```python
from build123d import *

# Parameters (mm, degrees)
BOSS_EXTRUDE1_DEPTH            = 1.6
F_2_2_2_2_DIAMETER_HOLE1_D     = 2.2
F_2_2_2_2_DIAMETER_HOLE1_DEPTH = 5
SKETCH9_R                      = 10
CUT_EXTRUDE4_DEPTH             = 2.6
SKETCH15_W                     = 83
SKETCH15_H                     = 2.5
CUT_EXTRUDE8_DEPTH             = 2.6
SKETCH37_W                     = 83
SKETCH37_H                     = 1.6
EXTRUDE1_DEPTH                 = 1.6
SKETCH38_W                     = 83
SKETCH38_H                     = 1.6
EXTRUDE2_DEPTH                 = 1.6
F_2_2_2_2_DIAMETER_HOLE4_D     = 2.2
F_2_2_2_2_DIAMETER_HOLE4_DEPTH = 1.6
SKETCH49_W                     = 0.2
SKETCH49_H                     = 100.7
EXTRUDE5_DEPTH                 = 2.6
SKETCH51_W                     = 10
SKETCH51_H                     = 10
CUT_EXTRUDE9_DEPTH             = 10
SKETCH52_W                     = 19
SKETCH52_H                     = 6.1
CUT_EXTRUDE10_DEPTH            = 2.6
SKETCH_2_R                     = 1.6
CUT_EXTRUDE_2_DEPTH            = 10
SKETCH_8_R                     = 0.3
CUT_EXTRUDE_3_DEPTH            = 10
SKETCH_9_R                     = 1.1
CUT_EXTRUDE_4_DEPTH            = 10
SKETCH_10_R                    = 2
CUT_EXTRUDE_5_DEPTH            = 0.01
SKETCH_11_R                    = 1.1
CUT_EXTRUDE_6_DEPTH            = 10


with BuildPart() as part:
    # Sketch1 → Boss-Extrude1 (new body)
    with BuildSketch(Plane(origin=(0, 0, 0), x_dir=(1, 0, 0), z_dir=(0, 1, 0))):
        Polygon((65.24, 0.272495156), (65.24, -46.437452638), (65.24, -63.637452638), (65.24, -70.137452638), (-17.76, -70.137452638), (-17.76, -63.637452638), (-17.76, -48.637452638), (-17.76, -45.78978272), (-17.76, 4.362547362), (-17.76, 21.562547362), (-17.76, 29.862547362), (65.24, 29.862547362), (65.24, 21.562547362), (65.24, 6.562547362), align=None)
    extrude(amount=BOSS_EXTRUDE1_DEPTH)

    # Ø2.2 (2.2) Diameter Hole1
    with Locations(Plane(origin=(0, 1.6, 0), x_dir=(1, 0, 0), z_dir=(0, 1, 0))):
        with Locations((57.24, 27.862547362), (-9.76, 27.862547362)):
            Hole(F_2_2_2_2_DIAMETER_HOLE1_D / 2, depth=F_2_2_2_2_DIAMETER_HOLE1_DEPTH)

    # Sketch9 → Cut-Extrude4 (cut, through all)
    with BuildSketch(Plane(origin=(0, 0, 0), x_dir=(-1, 0, 0), z_dir=(0, -1, 0))):
        with Locations((-11.54, -6.137452638)):
            Circle(SKETCH9_R)
    extrude(amount=-CUT_EXTRUDE4_DEPTH, mode=Mode.SUBTRACT)

    # Sketch15 → Cut-Extrude8 (cut, through all)
    with BuildSketch(Plane.XZ):
        with Locations((23.74, 68.887452638)):
            Rectangle(SKETCH15_W, SKETCH15_H)
    extrude(amount=-CUT_EXTRUDE8_DEPTH, mode=Mode.SUBTRACT)

    # Sketch37 → Extrude1 (add)
    with BuildSketch(Plane(origin=(0, 0, -29.862547362), x_dir=(-1, 0, 0), z_dir=(0, 0, -1))):
        with Locations((-23.74, 0.8)):
            Rectangle(SKETCH37_W, SKETCH37_H)
    extrude(amount=EXTRUDE1_DEPTH)

    # Sketch38 → Extrude2 (add)
    with BuildSketch(Plane.XY.offset(67.637452638)):
        with Locations((23.74, 0.8)):
            Rectangle(SKETCH38_W, SKETCH38_H)
    extrude(amount=EXTRUDE2_DEPTH)

    # Ø2.2 (2.2) Diameter Hole4
    with Locations(Plane(origin=(0, 1.6, 0), x_dir=(1, 0, 0), z_dir=(0, 1, 0))):
        with Locations((-8.76, -66.137452638), (56.24, -66.137452638)):
            Hole(F_2_2_2_2_DIAMETER_HOLE4_D / 2, depth=F_2_2_2_2_DIAMETER_HOLE4_DEPTH)

    # Sketch49 → Extrude5 (cut, through all)
    with BuildSketch(Plane.XZ):
        with Locations((65.14, 18.887452638)):
            Rectangle(SKETCH49_W, SKETCH49_H)
        with Locations((-17.66, 18.887452638)):
            Rectangle(SKETCH49_W, SKETCH49_H)
    extrude(amount=-EXTRUDE5_DEPTH, mode=Mode.SUBTRACT)

    # Sketch51 → Cut-Extrude9 (cut)
    with BuildSketch(Plane.XZ):
        with Locations((39.54, 6.037452638)):
            Rectangle(SKETCH51_W, SKETCH51_H)
    extrude(amount=-CUT_EXTRUDE9_DEPTH, mode=Mode.SUBTRACT)

    # Sketch52 → Cut-Extrude10 (cut, through all)
    with BuildSketch(Plane.XZ):
        with Locations((23.74, -19.027547362)):
            Rectangle(SKETCH52_W, SKETCH52_H)
    extrude(amount=-CUT_EXTRUDE10_DEPTH, mode=Mode.SUBTRACT)

    # ｽｹｯﾁ2 → ｶｯﾄ - 押し出し2 (cut)
    with BuildSketch(Plane(origin=(0, 0, 0), x_dir=(-1, 0, 0), z_dir=(0, -1, 0))):
        with Locations((-54.04, -29.237452638)):
            Circle(SKETCH_2_R)
        with Locations((6.56, -29.237452638)):
            Circle(SKETCH_2_R)
        with Locations((-41.74, 19.462547362)):
            Circle(SKETCH_2_R)
        with Locations((-5.74, 19.462547362)):
            Circle(SKETCH_2_R)
    extrude(amount=-CUT_EXTRUDE_2_DEPTH, mode=Mode.SUBTRACT)

    # ｽｹｯﾁ8 → ｶｯﾄ - 押し出し3 (cut)
    with BuildSketch(Plane(origin=(0, 1.6, 0), x_dir=(1, 0, 0), z_dir=(0, 1, 0))):
        with Locations((27.54, -28.337452638)):
            Circle(SKETCH_8_R)
        with Locations((19.94, -28.337452638)):
            Circle(SKETCH_8_R)
    extrude(amount=-CUT_EXTRUDE_3_DEPTH, mode=Mode.SUBTRACT)

    # ｽｹｯﾁ9 → ｶｯﾄ - 押し出し4 (cut)
    with BuildSketch(Plane(origin=(0, 1.6, 0), x_dir=(1, 0, 0), z_dir=(0, 1, 0))):
        with Locations((30.04, -30.237452638)):
            Circle(SKETCH_9_R)
        with Locations((17.44, -30.237452638)):
            Circle(SKETCH_9_R)
    extrude(amount=-CUT_EXTRUDE_4_DEPTH, mode=Mode.SUBTRACT)

    # ｽｹｯﾁ10 → ｶｯﾄ - 押し出し5 (cut)
    with BuildSketch(Plane(origin=(0, 1.6, 0), x_dir=(1, 0, 0), z_dir=(0, 1, 0))):
        with Locations((30.04, -30.237452638)):
            Circle(SKETCH_10_R)
        with Locations((17.44, -30.237452638)):
            Circle(SKETCH_10_R)
    extrude(amount=-CUT_EXTRUDE_5_DEPTH, mode=Mode.SUBTRACT)

    # ｽｹｯﾁ11 → ｶｯﾄ - 押し出し6 (cut)
    with BuildSketch(Plane(origin=(0, 1.6, 0), x_dir=(1, 0, 0), z_dir=(0, 1, 0))):
        with Locations((-3.51, -11.037452638)):
            Circle(SKETCH_11_R)
        with Locations((-3.51, -17.037452638)):
            Circle(SKETCH_11_R)
    extrude(amount=-CUT_EXTRUDE_6_DEPTH, mode=Mode.SUBTRACT)


solid = part.part
```
CAD build for the part. Positions are in the model's coordinates, mm. Coordinates: 2 decimals unless noted, no trailing zeros. Order: outer loops, then holes, each group sorted by start corner. A loop starts at its lowest first (then second) coordinate and runs counter-clockwise, first axis right, second up. Notation, with made-up numbers: M 78.5,-18.75 L 133.5,-18.75 A15 cw 133.5,-4.75 Z; hole C -14,27 d8. An arc over 180 degrees is marked long. Write each question's results on one line, items separated by ' | '. Start each with the question number.
Q1. Flat gauge pins, fed straight in: P1, Ø2, axis at x = -3.51, z = 11.04, coming from the -Y side; P2, Ø3.5, axis at x = 17.44, z = 30.24, coming from the +Y side. Where does each tip first touch, or does it go through?
Q2. Cut at B-B (y = 0.25). Count the separate pieces of the cut face and the enclosed holes in it, then the cut area to 3 significant figures.
Q3. Cut at C-C (x = -6.56). List the corners of the cut face in (y, z), then the cut area to 3 significant figures.
Q4. Drill centre lines: probe 1 along X at (y, z) = (0.65, 6.5); probe 2 along Z at (x, y) = (41.74, 0.9); probe 3 along Z at (x, y) = (5.74, 0.9). Where is each one in solid material? Low to high. Write a range as from..to.
Q5. Cut at A-A (x = 39). List the corners of the cut face in (y, z).
Q6. Pull direction Z, two halves, no side cores. Call faces 1 (the flat face through (31.3, 1.59, 30.2)), 2 (the cylindrical face through (17.2, 0.81, 31.31)): +Z half, -Z half, draft (parallel to the pull), parting line (faces both ways), or undercut.
Found:
1) P1: through | P2: y = 1.59
2) separate pieces: 1 | enclosed holes: 17 | area: 7,720 mm²
3) outline: M 0,-31.46 L 1.6,-31.46 L 1.6,27.64 L 0,27.64 Z; M 0,30.84 L 1.6,30.84 L 1.6,69.24 L 0,69.24 Z | area: 156 mm²
4) probe 1: -17.56..1.55, 21.53..34.54, 44.54..65.04 | probe 2: -31.46..-21.06, -17.86..1.04, 11.04..69.24 | probe 3: -31.46..-21.06, -17.86..-2.01, 14.28..69.24
5) outline: M 0,-31.46 L 1.6,-31.46 L 1.6,1.04 L 0,1.04 Z; M 0,11.04 L 1.6,11.04 L 1.6,69.24 L 0,69.24 Z
6) face 1: draft | face 2: undercut
